Geometry: see drawing. Coordinates: mm, zero at the bounding-box minimum. Give positions to 0.01 mm unless a question says otherwise; leave off trailing zeros. Use a Markdown table: item, result. Add a question column.
1) Pin query (flat end, axial travel): pin 1 (1.5 mm diameter, centred on x = 6.5, z = 4.5, fed in from +Y); pin 2 (4 mm diameter, centred on x = 2, y = 22, fed in from -Z). Return the tip coordinate at first contact, or that it passes through.
2) Section A-A on x = 4. State how many separate pieces and enclosed holes the cut face has, then the cut area to 3 significant figures.
3) Draft query along X for the marked faces 1, 2, 3 and 4. Return one class per face: +X half, -X half, draft (parallel to the pull), parting line (faces both ways), or undercut.
4) Line query: line 1 (Y direction, x = 4.5, z = 9.5) (1 decimal); line 2 (Y direction, x = 3.75, z = 6) (1 decimal); line 3 (Z direction, x = 6.75, y = 3). Output: solid intervals per line, ascending.
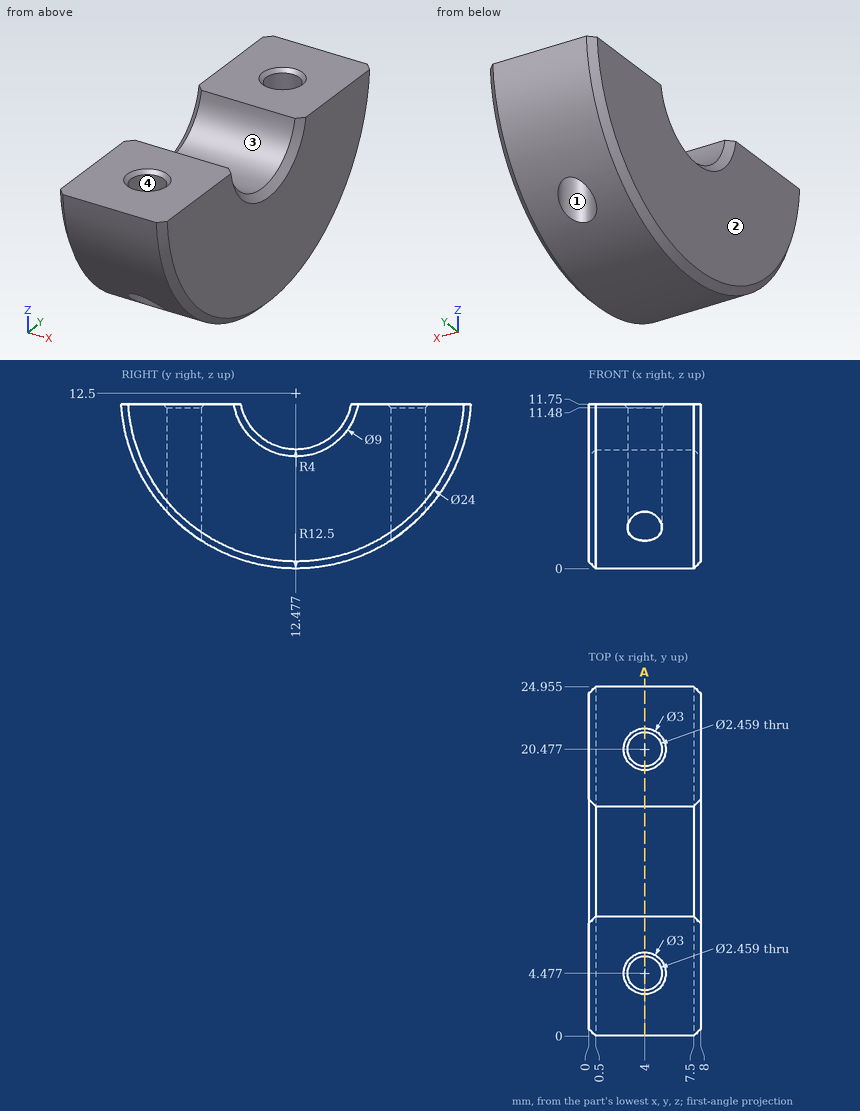
Found:
| question | item | result |
|---|---|---|
| 1 | pin 1 | y = 22.66 |
| 1 | pin 2 | z = 2.52 |
| 2 | separate pieces | 3 |
| 2 | enclosed holes | 0 |
| 2 | area | 164 mm² |
| 3 | face 1 | undercut |
| 3 | face 2 | -X half |
| 3 | face 3 | draft |
| 3 | face 4 | undercut |
| 4 | line 1 | 0.3 to 3.4, 5.6 to 9.8, 15.1 to 19.4, 21.6 to 24.6 |
| 4 | line 2 | 1.8 to 3.3, 5.7 to 19.3, 21.7 to 23.2 |
| 4 | line 3 | 4.35 to 11.75 |
